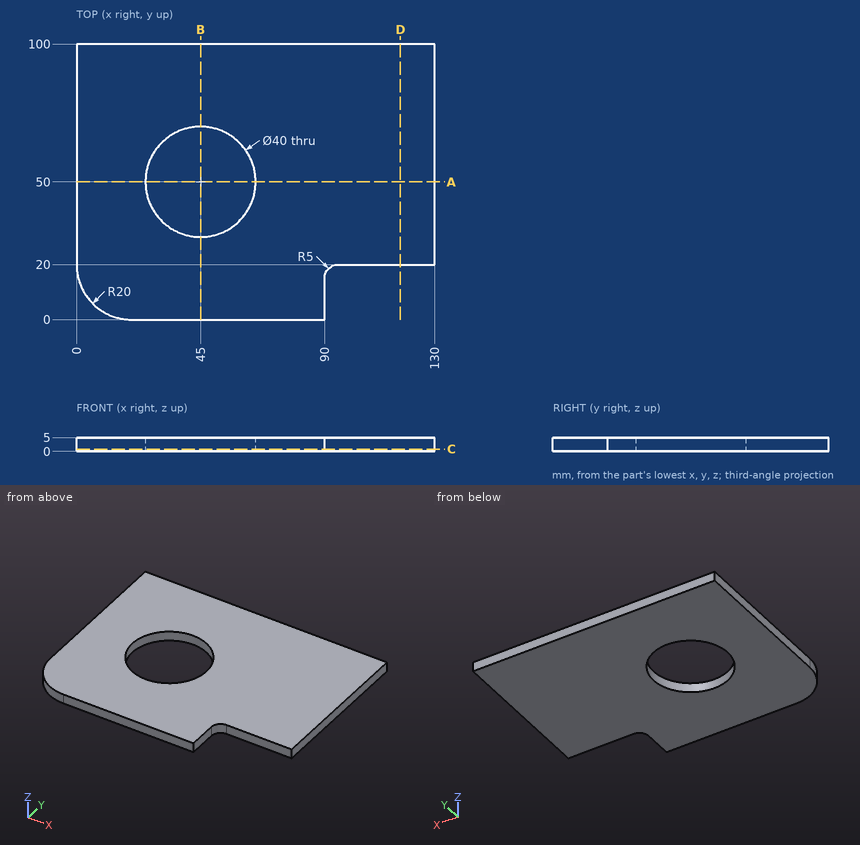
Input: dimensioned drawing with shaded views. Units: mm. Origin: part minimum x, y, z. Coordinates: 2 decimals unless noted, no trailing zeros. Loops run counter-clockwise (first coordinate to the right, second up) from the corner with the lowest first, then second, coordinate; pieces in that order, holes last. Notation, with made-up numbers: M 89,34.25 L 116,34.25 A17 ccw 116,47.25 Z; hole C -2,32.5 d6. An arc over 180 degrees is marked long. One line per item, written item: value. Start each with the question number.
1) Material intervals for L1, parallel to Y at x = 45, z = 2.6; L2, parallel to Y at x = 102.5, z = 2.6; L3, parallel to Y at x = 52, z = 3.55 (3 decimals), sorted ascending. Write a range as from..to.
2) Cut plane B-B (x = 45). Return loops of the section in (y, z).
3) Cut plane C-C (z = 0.85). Return loops of the section in (x, y), then the cut area to 3 significant figures.
4) Cut plane A-A (y = 50). Return loops of the section in (x, z).
5) Cut plane D-D (x = 117.5). Return loops of the section in (y, z), then the cut area to 3 significant figures.
6) Pin query (flat end, axial travel): P1, Ø1, axis at x = 104, z = 1, coming from the -Y side. Return the tip coordinate at first contact, or that it passes through.
Evaluation:
1. L1: 0..30, 70..100
1. L2: 20..100
1. L3: 0..31.265, 68.735..100
2. outline: M 0,0 L 30,0 L 30,5 L 0,5 Z; M 70,0 L 100,0 L 100,5 L 70,5 Z
3. outline: M 0,20 A20 ccw 20,0 L 90,0 L 90,15 A5 cw 95,20 L 130,20 L 130,100 L 0,100 Z; hole C 45,50 d40
3. area: 10,900 mm^2
4. outline: M 0,0 L 25,0 L 25,5 L 0,5 Z; M 65,0 L 130,0 L 130,5 L 65,5 Z
5. outline: M 20,0 L 100,0 L 100,5 L 20,5 Z
5. area: 400 mm^2
6. P1: y = 20
